Study the drawing (mm; zero at the part's minimum x, y, z) and answer. A direction names the side the tool comes from. Round coordinates to 2 decimals unless told otherwise and drop trailing zeros. Write each loop counter-clockwise with the first axis right and the second up, starting at its lowest first coordinate (ties: lowest second). Pieces come first, ordered by that corner, then holes. Notation, with made-up numbers: M 14.5,-9.75 L 27.5,-9.75 A20 cw 27.5,-5.75 Z; hole C -26.75,8.25 d3. An arc over 180 degrees is marked long. Write each question's results on one line, items separated by ' | '.
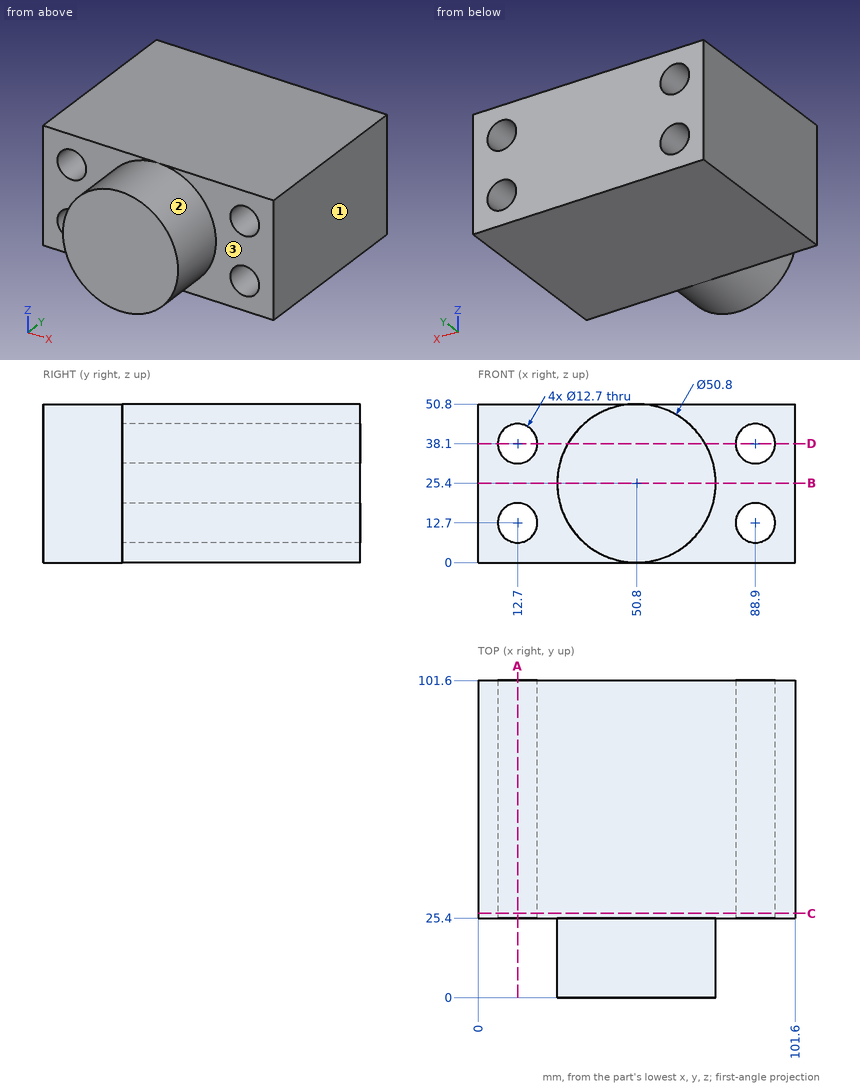
1) A tool of negligible diameter and unlimited length cuts with its end or side. For the marked faces 1, 2 and 3, from which of +Z, -Z, +X, -X, +Y, -Y can it reach the whole face along a straight path? Write none if from no direction.
Return value:
face 1: +Z, -Z, +X, +Y, -Y | face 2: -Y | face 3: +X, -Y
2) Section B-B (z = 25.4) is taken. Determine the outline of the cut face in (x, y), then the cut area to 3 significant figures.
Return value:
outline: M 0,25.4 L 25.4,25.4 L 25.4,0 L 76.2,0 L 76.2,25.4 L 101.6,25.4 L 101.6,101.6 L 0,101.6 Z | area: 9,030 mm²
3) Each of these flat-tipped pins is pushed along its axis until it touches: pin 1 (5 mm diameter, centred on x = 87.5, z = 19.5, fed in from -Y); pin 2 (4 mm diameter, centred on y = 13, z = 43, fed in from +X). Where does it stop, or does it pass through?
Return value:
pin 1: y = 25.4 | pin 2: x = 70.84
4) Section D-D (z = 38.1) is taken. Determine the outline of the cut face in (x, y).
Return value:
outline: M 0,25.4 L 6.35,25.4 L 6.35,101.6 L 0,101.6 Z; M 19.05,25.4 L 28.8,25.4 L 28.8,0 L 72.8,0 L 72.8,25.4 L 82.55,25.4 L 82.55,101.6 L 19.05,101.6 Z; M 95.25,25.4 L 101.6,25.4 L 101.6,101.6 L 95.25,101.6 Z
5) Section A-A (x = 12.7) is taken. Determine the outline of the cut face in (y, z), then the cut area to 3 significant figures.
Return value:
outline: M 25.4,0 L 101.6,0 L 101.6,6.35 L 25.4,6.35 Z; M 25.4,19.05 L 101.6,19.05 L 101.6,31.75 L 25.4,31.75 Z; M 25.4,44.45 L 101.6,44.45 L 101.6,50.8 L 25.4,50.8 Z | area: 1,940 mm²
6) Section C-C (y = 27) is taken. Determine the outline of the cut face in (x, z).
Return value:
outline: M 0,0 L 101.6,0 L 101.6,50.8 L 0,50.8 Z; hole C 12.7,12.7 d12.7; hole C 12.7,38.1 d12.7; hole C 88.9,12.7 d12.7; hole C 88.9,38.1 d12.7
7) Find the intervals of material crossed by line 1 (Z direction, x = 88.9, y = 48.5); line 2 (X direction, y = 73, z = 11); line 3 (X direction, y = 62, z = 7), in increasing order.
Return value:
line 1: 0 to 6.35, 19.05 to 31.75, 44.45 to 50.8 | line 2: 0 to 6.58, 18.82 to 82.78, 95.02 to 101.6 | line 3: 0 to 9.9, 15.5 to 86.1, 91.7 to 101.6
